Work out the finished part from the listing and answer in its coordinate system (mm). A direction names the side the tool comes from. Round coordinates to 2 decimals unless told otherwise and drop trailing zeros. Write each loop counter-clockwise with the first axis right and the second up, starting at its lowest first coordinate (ties: lowest second). Pieces come first, ordered by that corner, then holes. Notation, with made-up numbers: (88.5, 27.25) -> (108.5, 27.25) arc R27 cw to (108.5, 61.25) -> close; hole circle Ø7 at (80, 27). An arc over 180 degrees is marked (long way). One line per item, written item: value.
Autodesk Inventor part; units mm, degrees
ref_plane "Work Plane1" through (0, 15, 0) normal (0, 1, 0) x (-1, 0, 0)
ref_plane "YZ Plane" through (0, 0, 0) normal (1, 0, 0) x (0, 1, 0)
ref_plane "XY Plane" through (0, 0, 0) normal (0, 0, 1) x (1, 0, 0)
sketch "Sketch1" plane through (0, 0, 0) normal (0, 0, 1) x (1, 0, 0)
  line L0 (0, 0) -> (0, 15)
  line L1 (0, 0) -> (15, 0)
  arc A0 (15, 0) -> (0, 15) centre (0, 0) ccw
  line L2 (0, -3.6213) -> (0, 21.7279)
  dimension "d2" = 15
revolve "Revolution1" add sketch "Sketch1" angle 360 about axis through (0, -10, 0) along (0, 1, 0)
ref_plane "Work Plane1" through (0, 15, 0) normal (0, 1, 0) x (-1, 0, 0)
sketch "Sketch2" plane through (0, 15, 0) normal (0, 1, 0) x (-1, 0, 0)
  point P0 (0, 0)
  point P1 (0, 0)
hole "Hole1" at (0, 15, 0) direction (0, -1, 0) diameter 4.5 end through all counterbore diameter 8 counterbore depth 4
shell "Shell1" thickness 2 removed faces 1 at (10.5992, 0, 1.287)
sketch "Sketch3" plane through (0, 0, 0) normal (0, -1, 0) x (1, 0, 0)
  circle A0 centre (0, 0) radius 4.25
  circle A1 centre (0, 0) radius 2.25
extrude "Extrusion1" cut sketch "Sketch3" against normal blind 9
properties part number "Ball_Upper Half" material "Nylon 6/6"
(1) Find section D-D on y = 12.25. Give the vertices of the cut face in (x, z), plus the area to 3 significant figures.
Reported:
outline: circle Ø17.31 at (0, 0); hole circle Ø8 at (0, 0)
area: 185 mm2
(2) Find section A-A on z = 0. Give the vertices of the cut face in (x, y), plus the area to 3 significant figures.
Reported:
outline: (-15, 0) -> (-13, 0) arc R13 cw to (-6, 11.53) -> (-6, 9) -> (-2.25, 9) -> (-2.25, 11) -> (-4, 11) -> (-4, 14.46) arc R15 ccw to start; (2.25, 9) -> (6, 9) -> (6, 11.53) arc R13 cw to (13, 0) -> (15, 0) arc R15 ccw to (4, 14.46) -> (4, 11) -> (2.25, 11) -> close
area: 90.7 mm2
(3) Find section B-B on x = 1.5. Give the vertices of the cut face in (y, z).
Reported:
outline: (0, -14.92) arc R14.92 ccw to (14.46, -3.71) -> (11, -3.71) -> (11, -1.68) -> (9, -1.68) -> (9, -5.81) -> (11.53, -5.81) arc R12.91 cw to (0, -12.91) -> close; (0, 12.91) arc R12.91 cw to (11.53, 5.81) -> (9, 5.81) -> (9, 1.68) -> (11, 1.68) -> (11, 3.71) -> (14.46, 3.71) arc R14.92 ccw to (0, 14.92) -> close
(4) Consider probe 1 along X at (y, z) = (9.9, 0); probe 2 along Z at (x, y) = (0, 10.45); probe 3 along X at (y, z) = (10.75, -1.5). Determine where each line is inside the solid, lowest interval first.
Reported:
probe 1: x = -11.27 to -8.43, -6 to -2.25, 2.25 to 6, 8.43 to 11.27
probe 2: z = -10.76 to -7.73, -6 to -2.25, 2.25 to 6, 7.73 to 10.76
probe 3: x = -10.35 to -7.15, -5.81 to -1.68, 1.68 to 5.81, 7.15 to 10.35
(5) Flat-ended cylindrical pins translate along their axes: pin 1 Ø1.5 at (y, z) = (5, 4) entering from +X; pin 2 Ø4 at (x, z) = (0, 1) entering from +Y; pin 3 Ø13 at (x, z) = (0, 0) entering from -Y. Find the tip coordinate at first contact, or state that the pin passes through.
Reported:
pin 1: stops at x = 13.89
pin 2: stops at y = 11
pin 3: stops at y = 9
(6) A tool of negligible diameter and unlimited length cuts with its end or side. For faces 1 (the face through (-1.802, 10.249, 5.723)), 2 (the face through (3.905, 12.704, -0.867)), 3 (the face through (-2.23, 9.99, -0.29)), from which of +Z, -Z, +X, -X, +Y, -Y can it reach the whole face along a straight path? Write none if from no direction.
Reported:
face 1: -Y
face 2: +Y
face 3: +Y, -Y
(7) Find section C-C on z = -3.5. Give the vertices of the cut face in (x, y).
Reported:
outline: (-14.59, 0) -> (-12.52, 0) arc R12.52 cw to (-4.87, 11.53) -> (-4.87, 9) -> (4.87, 9) -> (4.87, 11.53) arc R12.52 cw to (12.52, 0) -> (14.59, 0) arc R14.59 ccw to (1.94, 14.46) -> (1.94, 11) -> (-1.94, 11) -> (-1.94, 14.46) arc R14.59 ccw to start
